Autodesk Inventor part; units mm, degrees
ref_plane "YZ Plane" through (0, 0, 0) normal (1, 0, 0) x (0, 1, 0)
ref_plane "XZ Plane" through (0, 0, 0) normal (0, 1, 0) x (-1, 0, 0)
ref_plane "XY Plane" through (0, 0, 0) normal (0, 0, 1) x (1, 0, 0)
sketch "Sketch1" plane through (0, 0, 0) normal (1, 0, 0) x (0, 1, 0)
  line L0 (412.75, 0) -> (412.75, 25.4)
  line L1 (412.75, 25.4) -> (488.95, 25.4)
  line L2 (488.95, 25.4) -> (488.95, -17.378)
  line L3 (488.95, -17.378) -> (476.25, -19.05)
  line L4 (476.25, -19.05) -> (476.25, -53.34)
  line L5 (476.25, -53.34) -> (488.95, -56.0974)
  line L6 (488.95, -56.0974) -> (488.95, -131.7625)
  line L7 (0, -218.44) -> (0, 66.04)
  line L8 (457.2, -144.4625) -> (457.2, -169.2731)
  line L9 (457.2, -169.2731) -> (446.0875, -177.8)
  line L10 (446.0875, -177.8) -> (444.5, -177.8)
  line L11 (444.5, -177.8) -> (444.5, -144.4625)
  arc A0 (425.45, -6.35) -> (419.1, 0) centre (419.1, -6.35) ccw
  line L12 (419.1, 0) -> (412.75, 0)
  arc A1 (469.9, -131.7625) -> (457.2, -144.4625) centre (469.9, -144.4625) ccw
  line L13 (425.45, -131.7625) -> (431.8, -131.7625)
  arc A2 (444.5, -144.4625) -> (431.8, -131.7625) centre (431.8, -144.4625) ccw
  line L14 (425.45, -131.7625) -> (425.45, -6.35)
  line L15 (488.95, -131.7625) -> (469.9, -131.7625)
  point P0 (0, 0)
  dimension "d0" = 412.75
  dimension "d5" = 25.4
  dimension "d13" = 476.25
  dimension "d14" = 488.95
  dimension "d16" = 44.45
  dimension "d17" = 34.29
  dimension "d18" = 7.5
  dimension "d19" = 12.25
  dimension "d32" = 457.2
  dimension "d33" = 11.1125
  dimension "d35" = 1.5875
  dimension "d36" = 6.35
  dimension "d38" = 203.2
  dimension "d44" = 12.7
  dimension "d46" = 37.5
  dimension "d47" = 12.7
  dimension "d48" = 425.45
  dimension "d49" = 157.1625
revolve "Revolution1" add sketch "Sketch1" angle 360 about axis through (0, 0, -10) along (0, 0, 1)
chamfer "Chamfer2" distance 0.7937 angle 45 1 edges at (0, -412.75, 0)
equation "\"d47\" = d44"
properties part number "A1-19027-100-03 36in Type B victaulic ring" material "Steel, Mild"
Can you work these out from the model? Positions are in its coordinate system, mm. A direction names the side the tool comes from. Coordinates: 2 decimals unless noted, no trailing zeros. Loops run counter-clockwise (first coordinate to the right, second up) from the corner with the lowest first, then second, coordinate; pieces in that order, holes last. Notation, with made-up numbers: M -5,-8.5 L 9,-8.5 A23 ccw 9,22.5 Z; hole C 72,6 d2. An arc over 180 degrees is marked long. Put each result on its own line as item: value. Start each with the question number.
(1) Which directions (+Z, -Z, +X, -X, +Y, -Y) give clear straight access to the entire face, cutting with the end or side of a thin tool? Please do faces 5 (the face through (251, -328, 25.4)), 6 (the face through (143.291, 455.015, -53.512)), 7 (the face through (-401, -256, -131.762)).
(2) Imagine slicing it at A-A on z = -72. List the corners of the cut face in (x, y) for me.
(3) We'd pull the mould along Z, two halves only. Please class faces 1 (the face through (-289.791, -377.936, -36.435)), 2 (the face through (436.158, -96.854, -177.267)), 3 (the face through (251.152, -327.544, 13.269)), 4 (the face through (290.274, -378.566, -18.945)): +Z half, -Z half, draft (parallel to the pull), parting line (faces both ways), or undercut.
(4) I need wall thicknesses on probe 1 along X at (y, z) = (0, 15); probe 2 along X at (y, z) = (0, -164); probe 3 along Y at (x, z) = (78, -167). Which ranges of each line are inside material? Lowest first, please.
(5) Will these pins go through, and if not, where does the flat tip stop? pin 1 Ø8 at (x, z) = (356.5, -72) entering from +Y; pin 2 Ø2 at (y, z) = (95.5, -48) entering from -X; pin 3 Ø1.5 at (y, z) = (105.5, -68.5) entering from -X.
Worked answers:
1. face 5: +Z, +X, -X, +Y, -Y
1. face 6: none
1. face 7: -Z
2. outline: C 0,0 d977.9; hole C 0,0 d850.9
3. face 1: undercut
3. face 2: -Z half
3. face 3: draft
3. face 4: undercut
4. probe 1: x = -488.95 to -412.75, 412.75 to 488.95
4. probe 2: x = -457.2 to -444.5, 444.5 to 457.2
4. probe 3: y = -450.5 to -437.6, 437.6 to 450.5
5. pin 1: stops at y = 338.84
5. pin 2: stops at x = -466.78
5. pin 3: stops at x = -477.6
